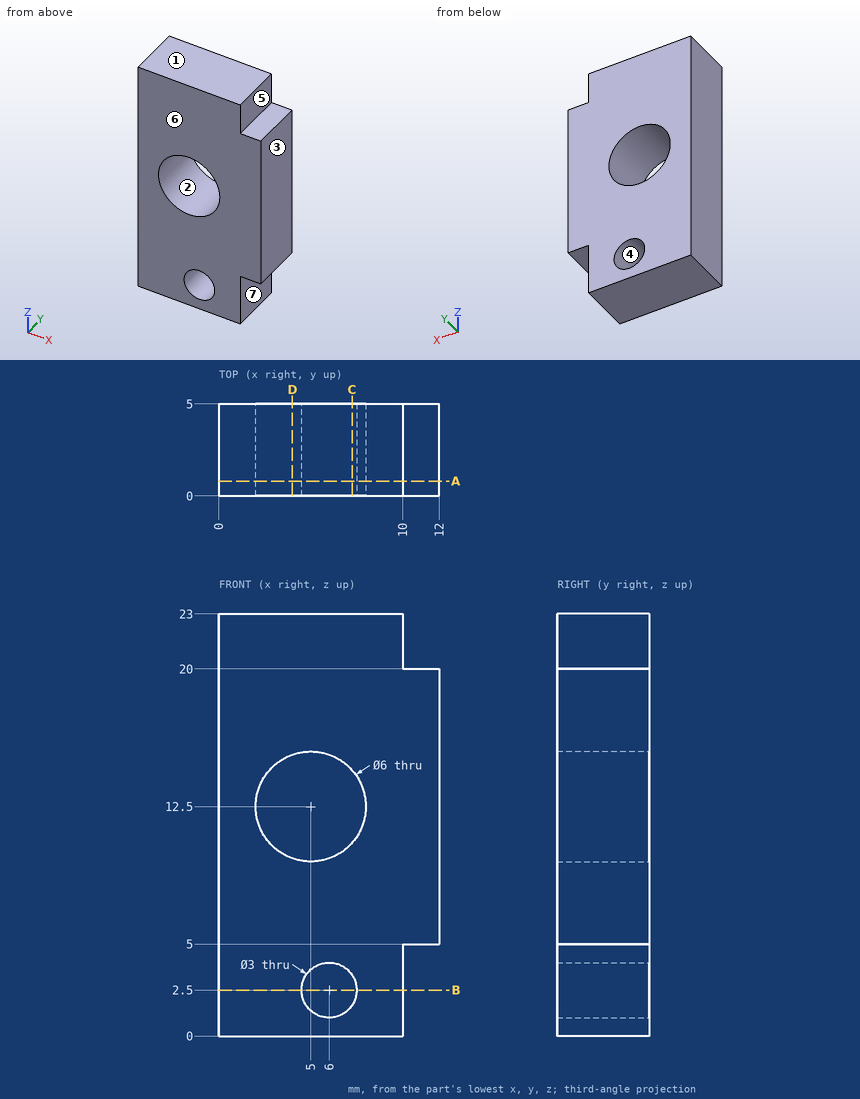
The figure shows three views and two pictorial views of one solid part (mm, origin at its lowest corner). Answer the questions. A direction names the side the tool comes from. Round coordinates to 2 decimals unless told otherwise and drop trailing zeros. Write each loop counter-clockwise with the first axis right and the second up, starting at its lowest first coordinate (ties: lowest second). Pieces come first, ordered by that corner, then holes. Notation, with made-up numbers: (72, 32) - (114, 32) arc R21 cw to (114, 46) - close; hole circle Ø6 at (20.5, 43). An arc over 180 degrees is marked (long way). One line per question, with ' | ' between items. Start each with the question number.
1. Section D-D (x = 4) is taken. Determine the outline of the cut face in (y, z), and give its area (3 significant figures).
2. Section A-A (y = 0.8) is taken. Determine the outline of the cut face in (x, z).
3. Find the intervals of material crossed by probe 1 along Z at (x, y) = (6, 2.15); probe 2 along Z at (x, y) = (5, 3); probe 3 along X at (y, z) = (2.6, 2.5), in increasing order. Write a range as [from, to].
4. For the marked faces 5, 6 and 7, determine the directions among +Z, -Z, +X, -X, +Y, -Y from which every point of the face is accessible in a straight line to the end or side of a thin tool.
5. Each of these flat-tipped pins is pushed along its axis until it touches: pin 1 (0.6 mm diameter, centred on x = 11, y = 3, fed in from +Z); pin 2 (2 mm diameter, centred on x = 6, z = 18, fed in from -Y); pin 3 (2.5 mm diameter, centred on x = 6, z = 2.5, fed in from +Y); pin 4 (2.5 mm diameter, centred on y = 3.5, z = 21.5, fed in from +X). Where does it stop, or does it pass through?
6. Section B-B (z = 2.5) is taken. Determine the outline of the cut face in (x, y), and give its area (3 significant figures).
7. For a pull along X with two mould halves and no side action, classify the marked faces 1, 2, 3 and 4 as +X half, -X half, draft (parallel to the pull), parting line (faces both ways), or undercut.
8. Section C-C (x = 7.25) is taken. Determine the outline of the cut face in (y, z), and give its area (3 significant figures).
Filled in:
1) outline: (0, 0) - (5, 0) - (5, 9.67) - (0, 9.67) - close; (0, 15.33) - (5, 15.33) - (5, 23) - (0, 23) - close | area: 86.7 mm²
2) outline: (0, 0) - (10, 0) - (10, 5) - (12, 5) - (12, 20) - (10, 20) - (10, 23) - (0, 23) - close; hole circle Ø6 at (5, 12.5); hole circle Ø3 at (6, 2.5)
3) probe 1: [0, 1], [4, 9.67], [15.33, 23] | probe 2: [0, 1.38], [3.62, 9.5], [15.5, 23] | probe 3: [0, 4.5], [7.5, 10]
4) face 5: +Z, +X, +Y, -Y | face 6: +Z, -Z, +X, -X, -Y | face 7: -Z, +X, +Y, -Y
5) pin 1: z = 20 | pin 2: y = 0 | pin 3: through | pin 4: x = 10
6) outline: (0, 0) - (4.5, 0) - (4.5, 5) - (0, 5) - close; (7.5, 0) - (10, 0) - (10, 5) - (7.5, 5) - close | area: 35.0 mm²
7) face 1: draft | face 2: undercut | face 3: +X half | face 4: undercut
8) outline: (0, 0) - (5, 0) - (5, 1.67) - (0, 1.67) - close; (0, 3.33) - (5, 3.33) - (5, 10.52) - (0, 10.52) - close; (0, 14.48) - (5, 14.48) - (5, 23) - (0, 23) - close | area: 86.9 mm²
